Could you check a few things on this model? Use its own coordinates, in mm. A direction names the side the tool comes from. Give positions to 0.01 mm unless a question says otherwise; leave off trailing zeros. Write each loop counter-clockwise with the first axis right and the second up, starting at its lowest first coordinate (ties: lowest second). Pieces come first, ordered by that corner, then holes. Notation, with made-up numbers: (42.5, -30) -> (92.5, -30) arc R5 cw to (92.5, -26) -> close; hole circle Ø11 at (13, -22). An arc over 180 degrees is marked (long way). Write item = value, one per line. Start each with the question number.
Autodesk Inventor part; units mm, degrees
ref_plane "Work Plane2" through (-32.45, 25, -313.9) normal (0, 0, -1) x (-1, 0, 0)
ref_plane "YZ Plane" through (0, 0, 0) normal (1, 0, 0) x (0, 1, 0)
ref_plane "XZ Plane" through (0, 0, 0) normal (0, 1, 0) x (-1, 0, 0)
sketch "Sketch1" plane through (0, 0, 0) normal (0, 1, 0) x (-1, 0, 0)
  line L0 (0, 0) -> (90, 0)
  line L1 (90, 0) -> (90, -500)
  line L2 (90, -500) -> (0, -500)
  line L3 (0, -500) -> (0, 0)
  dimension "d0" = 90
  dimension "d1" = 500
extrude "Extrusion1" add sketch "Sketch1" along normal blind 25
sketch "Sketch6" plane through (0, 25, 0) normal (0, 1, 0) x (1, 0, 0)
  line L0 (-57.55, 311.9) -> (-32.45, 311.9)
  line L1 (-32.45, 311.9) -> (-32.45, 400)
  line L2 (-32.45, 400) -> (-57.55, 400)
  line L3 (-57.55, 400) -> (-57.55, 311.9)
  line L4 (-90, 500) -> (-90, 0)
  line L5 (0, 500) -> (-90, 500)
  point P0 (0, 0)
  dimension "d36" = 25.1
  dimension "d37" = 88.1
  dimension "d38" = 32.45
  dimension "d39" = 100
extrude "Extrusion6" cut sketch "Sketch6" against normal blind 20
sketch "Sketch7" plane through (-32.45, 25, -311.9) normal (0, 0, -1) x (-1, 0, 0)
  line L0 (0, 0) -> (25.1, 0)
  line L1 (0, 0) -> (0, -20)
  line L2 (0, -20) -> (25.1, -20)
  line L3 (25.1, 0) -> (25.1, -20)
  line L4 (0, -4) -> (25.1, -4)
  line L5 (25.1, -4) -> (25.1, -23)
  line L6 (0, -4) -> (0, -23)
  line L7 (25.1, -23) -> (0, -23)
  point P0 (-32.45, -25)
  dimension "d42" = 16
  dimension "d43" = 19
  dimension "d44" = 19
ref_plane "Work Plane2" through (-32.45, 25, -313.9) normal (0, 0, -1) x (-1, 0, 0)
sketch "Sketch9" plane through (-32.45, 25, -313.9) normal (0, 0, -1) x (-1, 0, 0)
  line L0 (25.1, -4) -> (25.1, -23)
  line L1 (0, 0) -> (0, -20)
  line L2 (25.1, -23) -> (0, -23)
  line L3 (0, -23) -> (0, -4)
  line L4 (0, 0) -> (25.1, 0)
  line L5 (25.1, -4) -> (25.1, 0)
  line L6 (0, 0) -> (25.1, 0)
  line L7 (0, 0) -> (0, -4)
  line L8 (25.1, -3) -> (0, -3)
  point P0 (-32.45, -25)
  dimension "d97" = 3
extrude "Extrusion9" cut sketch "Sketch9" against normal blind 22 contours L0 L2 L3 L1 L8 L5
sketch "Sketch12" plane through (0, 25, 0) normal (0, 1, 0) x (1, 0, 0)
  line L0 (-17.5, 480) -> (-72.5, 480)
  line L1 (-72.5, 480) -> (-72.5, 425)
  line L2 (-72.5, 425) -> (-17.5, 425)
  line L3 (-17.5, 425) -> (-17.5, 480)
  line L4 (0, 0) -> (0, 500)
  line L5 (-32.45, 311.9) -> (-57.55, 311.9)
  line L6 (0, 500) -> (-90, 500)
  dimension "d57" = 55
  dimension "d58" = 55
  dimension "d59" = 17.5
  dimension "d100" = 20
extrude "Extrusion11" cut sketch "Sketch12" against normal blind 30
sketch "Sketch13" plane through (0, 0, 0) normal (0, -1, 0) x (1, 0, 0)
  line L0 (-72.5, -425) -> (-17.5, -425)
  line L1 (-17.5, -425) -> (-17.5, -480)
  line L2 (-17.5, -480) -> (-72.5, -480)
  line L3 (-72.5, -480) -> (-72.5, -425)
  line L4 (-7.5, -490) -> (-7.5, -415)
  line L5 (-7.5, -415) -> (-82.5, -415)
  line L6 (-82.5, -415) -> (-82.5, -490)
  line L7 (-82.5, -490) -> (-7.5, -490)
  point P0 (0, 0)
  dimension "d68" = 10
extrude "Extrusion12" cut sketch "Sketch13" against normal blind 14
sketch "Sketch14" plane through (0, 25, 0) normal (0, 1, 0) x (1, 0, 0)
  line L0 (-72.5, 425) -> (-72.5, 480)
  line L1 (-17.5, 425) -> (-72.5, 425)
  line L2 (-17.5, 480) -> (-17.5, 425)
  line L3 (-72.5, 480) -> (-17.5, 480)
  line L4 (-75, 482.5) -> (-75, 422.5) construction
  line L5 (-75, 422.5) -> (-15, 422.5) construction
  line L6 (-15, 422.5) -> (-15, 482.5) construction
  line L7 (-15, 482.5) -> (-75, 482.5) construction
  circle A0 centre (-75, 422.5) radius 2.05
  circle A1 centre (-75, 482.5) radius 2.05
  circle A2 centre (-15, 482.5) radius 2.05
  circle A3 centre (-15, 422.5) radius 2.05
  point P0 (0, 0)
  dimension "d69" = 2.5
  dimension "d70" = 4.1
  dimension "d71" = 4.1
  dimension "d72" = 4.1
  dimension "d73" = 4.1
fillet "Fillet14" radius 5 4 edges at (-82.5, 7, -415) (-7.5, 7, -415) (-7.5, 7, -490) (-82.5, 7, -490)
fillet "Fillet15" radius 2 8 edges at (-8.9645, 0, -488.5355) (-45, 0, -490) (-81.0355, 0, -488.5355) (-82.5, 0, -452.5) (-81.0355, 0, -416.4645) (-45, 0, -415) (-8.9645, 0, -416.4645) (-7.5, 0, -452.5)
sketch "Sketch15" plane through (0, 0, 0) normal (0, -1, 0) x (1, 0, 0)
  line L0 (-57.55, -311.625) -> (-32.45, -311.625)
  line L1 (-32.45, -311.625) -> (-32.45, -261.625)
  line L2 (-32.45, -261.625) -> (-57.55, -261.625)
  line L3 (-57.55, -261.625) -> (-57.55, -311.625)
  line L4 (-90, 0) -> (-90, -500)
  line L5 (-90, -500) -> (0, -500)
  point P0 (0, 0)
  dimension "d81" = 25.1
  dimension "d82" = 50
  dimension "d83" = 32.45
  dimension "d84" = 188.375
extrude "Extrusion14" cut sketch "Sketch15" against normal blind 15
fillet "Fillet16" radius 2 1 edges at (-45, 15, -291.9)
fillet "Fillet17" radius 2 3 edges at (-32.45, 0, -286.625) (-57.55, 0, -286.625) (-45, 0, -311.625)
fillet "Fillet18" radius 5 3 edges at (0, 25, -250) (-45, 25, 0) (-45, 25, -500)
fillet "Fillet19" radius 15 4 edges at (-1.4645, 23.5355, -1.4645) (0, 10, 0) (-1.4645, 23.5355, -498.5355) (0, 10, -500)
sketch "Sketch22" plane through (-57.55, 2, -313.9) normal (0, 1, 0) x (1, 0, 0)
  line L0 (0, -2.275) -> (25.1, -2.275)
  line L1 (25.1, 0) -> (25.1, -2.275)
  line L2 (25.1, 0) -> (0, 0)
  line L3 (0, 0) -> (0, -2.275)
  point P0 (57.55, -313.9)
extrude "Extrusion18" cut sketch "Sketch22" against normal blind 6
sketch "Sketch23" plane through (0, 0, 0) normal (0, -1, 0) x (1, 0, 0)
  point P0 (0, 0)
sketch "Sketch24" plane through (0, 25, 0) normal (0, 1, 0) x (1, 0, 0)
  line L0 (-24.2952, 12.3012) -> (-24.2952, 52.9327) construction
  line L1 (-24.2952, 52.9327) -> (-73.6667, 52.9327) construction
  line L2 (-73.6667, 52.9327) -> (-73.6667, 12.3012) construction
  line L3 (-73.6667, 12.3012) -> (-24.2952, 12.3012) construction
  point P0 (0, 0)
extrude "Extrusion19" [suppressed]
sketch "Sketch25" plane through (0, 14, 0) normal (0, -1, 0) x (1, 0, 0)
  line L0 (-17.5, -480) -> (-17.5, -425)
  line L1 (-17.5, -425) -> (-72.5, -425)
  line L2 (-72.5, -480) -> (-17.5, -480)
  line L3 (-72.5, -425) -> (-72.5, -480)
  circle A0 centre (-75, -482.5) radius 2.05
  circle A1 centre (-15, -482.5) radius 2.05
  circle A2 centre (-15, -422.5) radius 2.05
  circle A3 centre (-75, -422.5) radius 2.05
  point P0 (0, 0)
extrude "Extrusion20" cut sketch "Sketch25" against normal blind 1 contours A0 | A1 | A2 | A3
properties part number "Hilla" material "Lauan, Meranti"
(1) We'd pull the mould along X, two halves only. Please class faces 1 (the flat face through (-82.5, 8, -452)), 2 (the flat face through (-45, 8, -490)), 3 (the flat face through (-53, 10, -500)), 4 (the cylindrical face through (-4.28, 9.86, -4.51)): released by +X, released by -X, zero draft, split by the parting line, or undercut.
(2) Imagine slicing it at A-A (x = -38). Please give me the cut outline in (y, z) (3 decimals), then the cut area to 3 significant figures.
(3) On a 3-axis mill with a long thin cutter (end or side, diameter ignored), from which of +Z, -Z, +X, -X, +Y, -Y can I reach the whole of each face in a straight line? I mean faces 5 (the flat face through (-47, 25, -247)), 6 (the flat face through (-32.45, 15, -332)), 7 (the flat face through (-45, 22, -302)), 8 (the flat face through (0, 10, -253)), 9 (the flat face through (-72.5, 20, -453)). Say none if no direction works.
(4) Imagine slicing it at B-B (z = -377). Please give me the cut outline in (x, y).
(5) If I drill on line 1 along Z through (x, y) = (-41, 8.75) (3 decimals); line 2 along X through (y, z) = (14.75, -482.5); line 3 along Z through (x, y) = (-75, 14.2), over which ranges is the centre line in solid material (lowest first)? Write a range as from..to.
(6) I'm going to push flat-ended pins straight in: pin 1 (5.5 mm diameter, centred on x = -15, z = -422.5, fed in from -Y); pin 2 (3.5 mm diameter, centred on x = -75, z = -482.5, fed in from -Y); pin 3 (7.5 mm diameter, centred on x = -44, z = -346.5, fed in from +Y). Where does each tip first touch, or does it pass through?
Answers below:
q1.face_1 = undercut
q1.face_2 = undercut
q1.face_3 = zero draft
q1.face_4 = released by +X
q2.outline = (0, -500) -> (20, -500) arc R5 ccw to (25, -495) -> (25, -480) -> (14, -480) -> (14, -490) -> (2, -490) arc R2 ccw to (0, -492) -> close; (0, -413) arc R2 ccw to (2, -415) -> (14, -415) -> (14, -425) -> (25, -425) -> (25, -400) -> (5, -400) -> (5, -313.9) -> (0, -313.9) -> close; (0, -261.625) -> (15, -261.625) -> (15, -289.9) arc R2 ccw to (17, -291.9) -> (22, -291.9) -> (22, -311.9) -> (25, -311.9) -> (25, -5) arc R5 ccw to (20, 0) -> (0, 0) -> close
q2.area = 8,170 mm^2
q3.face_5 = +Z, -Z, +X, -X, +Y
q3.face_6 = none
q3.face_7 = -Y
q3.face_8 = +Z, -Z, +X, +Y, -Y
q3.face_9 = +Y, -Y
q4.outline = (-90, 0) -> (0, 0) -> (0, 20) arc R5 ccw to (-5, 25) -> (-32.45, 25) -> (-32.45, 5) -> (-57.55, 5) -> (-57.55, 25) -> (-90, 25) -> close
q5.line_1 = -500..-490, -415..-400, -261.625..0
q5.line_2 = -90..-77.05, -72.95..-17.05, -12.95..0
q5.line_3 = -500..-484.55, -480.45..-424.55, -420.45..0
q6.pin_1 = 14
q6.pin_2 = 15
q6.pin_3 = 5
